Autodesk Inventor part; units mm, degrees
ref_plane "YZ Plane" through (0, 0, 0) normal (1, 0, 0) x (0, 1, 0)
ref_plane "XZ Plane" through (0, 0, 0) normal (0, 1, 0) x (-1, 0, 0)
ref_plane "XY Plane" through (0, 0, 0) normal (0, 0, 1) x (1, 0, 0)
sketch "Sketch1" plane through (0, 0, 0) normal (0, 1, 0) x (-1, 0, 0)
  line L0 (0, 0) -> (19.4, 0)
  line L1 (19.4, 0) -> (19.4, -19.4)
  line L2 (19.4, -19.4) -> (0, -19.4)
  line L3 (0, -19.4) -> (0, 0)
  dimension "d0" = 19.4
  dimension "d1" = 19.4
extrude "Extrusion1" add sketch "Sketch1" along normal blind 3
sketch "Sketch2" plane through (0, 3, 0) normal (0, 1, 0) x (1, 0, 0)
  line L0 (-18.55, 2.013) -> (-18.55, 5.188)
  line L1 (-18.55, 5.188) -> (-15.8004, 6.7755)
  line L2 (-15.8004, 6.7755) -> (-13.0507, 5.188)
  line L3 (-13.0507, 5.188) -> (-13.0507, 2.013)
  line L4 (-13.0507, 2.013) -> (-15.8004, 0.4255)
  line L5 (-15.8004, 0.4255) -> (-18.55, 2.013)
  line L6 (-19.4, 0) -> (0, 0)
  line L7 (-19.4, 19.4) -> (-19.4, 0)
  dimension "d4" = 3.175
  dimension "d5" = 3.175
  dimension "d7" = 3.175
  dimension "d8" = 3.175
  dimension "d9" = 3.175
  dimension "d10" = 3.175
  dimension "d11" = 120
  dimension "d12" = 120
  dimension "d13" = 2.013
  dimension "d14" = 0.85
extrude "Extrusion2" cut sketch "Sketch2" against normal blind 2
pattern_linear "Rectangular Pattern1" count 2 spacing 12.2 along (0, 0, -1) count 2 spacing 12.2 along (1, 0, 0) of "Extrusion2"
sketch "Sketch3" plane through (0, 1, 0) normal (0, 1, 0) x (1, 0, 0)
  circle A0 centre (-15.8, 3.6) radius 1.6
  line L0 (-19.4, 19.4) -> (-19.4, 0)
  line L1 (-19.4, 0) -> (0, 0)
  dimension "d23" = 3.2
  dimension "d24" = 3.6
  dimension "d25" = 3.6
extrude "Extrusion3" cut sketch "Sketch3" against normal through all
pattern_linear "Rectangular Pattern2" count 2 spacing 12.2 along (0, 0, -1) count 2 spacing 12.2 along (1, 0, 0) of "Extrusion3"
equation "\"d1\" = d0"
equation "\"d5\" = d4"
equation "\"d7\" = d5"
equation "\"d9\" = d7"
equation "\"d10\" = d4"
properties part number "BOUCHON"
Design review of the part built by this model. Coordinates are the model's own, in mm. A direction names the side the tool comes from. Round coordinates to 2 decimals unless told otherwise and drop trailing zeros. Write each loop counter-clockwise with the first axis right and the second up, starting at its lowest first coordinate (ties: lowest second). Pieces come first, ordered by that corner, then holes.
Item 1: Consider section C-C on x = -2.25. Give the boundary of the cut face in (y, z).
Item 2: Consider section B-B on y = 2.05. Give the boundary of the cut face in (x, z).
Item 3: Consider section D-D on x = -5.5. Give the boundary of the cut face in (y, z), and give its area (3 significant figures).
Item 4: For pin 1 Ø2.5 at (x, z) = (-15.5, -14.5) entering from +Y, flat-tipped, find the tip position at first contact; note if it passes through.
Item 5: Draft analysis for pull direction Z (two halves, no side actions). For faces 1 (the flat face through (-13.051, 2, -16)), 2 (the flat face through (-10, 1, -19.4)), 3 (the flat face through (-10, 0, -10)), state which applies: released by +Z, released by -Z, zero draft, split by the parting line, or undercut.
Item 6: For faces 4 (the cylindrical face through (-14.274, 0.507, -4.081)), 5 (the flat face through (-0.851, 2, -4)), list the 3-axis set-ups (+Z, -Z, +X, -X, +Y, -Y) from which the entire face can be reached by the end or side of a thin tool; tool diameter is ignored.
Item 7: Wall thickness on L1, parallel to X at y = 0.65, z = -15.8; L2, parallel to X at y = 1.9, z = -4.5: over which ranges is each line inside the solid? List them lowest first.
Item 8: Consider section A-A on z = -3.6. Give the boundary of the cut face in (x, y), and give its area (3 significant figures).
Check values:
1. outline: (0, -19.4) - (3, -19.4) - (3, -18.2) - (1, -18.2) - (1, -16.66) - (0, -16.66) - close; (0, -14.94) - (1, -14.94) - (1, -13.41) - (3, -13.41) - (3, -6) - (1, -6) - (1, -4.46) - (0, -4.46) - close; (0, -2.74) - (1, -2.74) - (1, -1.21) - (3, -1.21) - (3, 0) - (0, 0) - close
2. outline: (-19.4, -19.4) - (0, -19.4) - (0, 0) - (-19.4, 0) - close; hole (-18.55, -17.39) - (-15.8, -18.98) - (-13.05, -17.39) - (-13.05, -14.21) - (-15.8, -12.63) - (-18.55, -14.21) - close; hole (-18.55, -5.19) - (-15.8, -6.78) - (-13.05, -5.19) - (-13.05, -2.01) - (-15.8, -0.43) - (-18.55, -2.01) - close; hole (-6.35, -17.39) - (-3.6, -18.98) - (-0.85, -17.39) - (-0.85, -14.21) - (-3.6, -12.63) - (-6.35, -14.21) - close; hole (-6.35, -5.19) - (-3.6, -6.78) - (-0.85, -5.19) - (-0.85, -2.01) - (-3.6, -0.43) - (-6.35, -2.01) - close
3. outline: (0, -19.4) - (3, -19.4) - (3, -17.88) - (1, -17.88) - (1, -13.72) - (3, -13.72) - (3, -5.68) - (1, -5.68) - (1, -1.52) - (3, -1.52) - (3, 0) - (0, 0) - close
3. area: 41.6 mm2
4. pin 1: stops at y = 1
5. face 1: undercut
5. face 2: released by -Z
5. face 3: zero draft
6. face 4: +Y, -Y
6. face 5: +Y
7. L1: x = -19.4 to -17.4, -14.2 to -5.2, -2 to 0
7. L2: x = -19.4 to -18.55, -13.05 to -6.35, -0.85 to 0
8. outline: (-19.4, 0) - (-17.4, 0) - (-17.4, 1) - (-18.55, 1) - (-18.55, 3) - (-19.4, 3) - close; (-14.2, 0) - (-5.2, 0) - (-5.2, 1) - (-6.35, 1) - (-6.35, 3) - (-13.05, 3) - (-13.05, 1) - (-14.2, 1) - close; (-2, 0) - (0, 0) - (0, 3) - (-0.85, 3) - (-0.85, 1) - (-2, 1) - close
8. area: 29.8 mm2
